from build123d import *

# Parameters (mm, degrees)
F1_DEPTH  = 16
F2_W      = 70
F2_H      = 3
F3_DEPTH  = 2
F4_W      = 50
F4_H      = 14
F5_DEPTH  = 2
F6_R      = 1
F9_DEPTH  = 2
F11_DEPTH = 38.001
F13_D     = 4
F14_R     = 3
F14_R_2   = 2
F15_DEPTH = 5
F16_R     = 3


# Not quite as in the source:
# - a pattern or mirror of a feature is missing from the dataset's text; its kind, count and spacing are read off the source's solid


with BuildPart() as f1:
    # F0 (on Front) → F1 (new body)
    with BuildSketch(Plane.XZ):
        with BuildLine():
            Line((94, 9), (0, 9))
            ThreePointArc((0, 9), (-9, 0), (0, -9))
            Line((0, -9), (19, -9))
            ThreePointArc((19, -9), (21.9483530121, -9.9617807742), (23.7624383273, -12.4771141937))
            ThreePointArc((23.7624383273, -12.4771141937), (42.5404984663, -42.5461666629), (73.3918884835, -60.0091329916))
            ThreePointArc((73.3918884835, -60.0091329916), (79.2017940664, -60.9932244785), (84.0921252778, -64.2807919045))
            Line((84.0921252778, -64.2807919045), (85.6344375761, -63))
            ThreePointArc((85.6344375761, -63), (80.1625330731, -59.2251678092), (73.628769931, -58))
            ThreePointArc((73.628769931, -58), (43.8155502437, -40.9978046119), (25.6674136582, -11.8679598712))
            ThreePointArc((25.6674136582, -11.8679598712), (23.127694217, -8.3464930839), (19, -7))
            Line((19, -7), (0, -7))
            ThreePointArc((0, -7), (-7, 0), (0, 7))
            Line((0, 7), (94, 7))
            Line((94, 7), (94, 9))
        make_face()
    extrude(amount=F1_DEPTH)

    # F2 (on face) → F3 (join)
    with BuildSketch(Plane.XY.offset(9)):
        with Locations((59, -17.5)):
            Rectangle(F2_W, F2_H)
    extrude(amount=-F3_DEPTH)

    # F4 (on face) → F5 (join)
    with BuildSketch(Plane.XZ.offset(19)):
        with Locations((69, 2)):
            Rectangle(F4_W, F4_H)
    extrude(amount=-F5_DEPTH)

    # F6
    f6_edges = [f1.edges().sort_by_distance(p)[0] for p in [
        (69, -17, 7),
        (59, -19, 9),
    ]]
    fillet(f6_edges, radius=F6_R)

    # F7: F1 across plane


with BuildPart() as f1_1:
    add(f1.part)
    add(f1.part.mirror(Plane.XZ))

    # F8 (on face) → F9 (cut)
    with BuildSketch(Plane.XY.offset(9)):
        with BuildLine():
            Line((94, 12), (34, 12))
            ThreePointArc((34, 12), (22, 0), (34, -12))
            Line((34, -12), (94, -12))
            Line((94, -12), (94, 12))
        make_face()
    extrude(amount=-F9_DEPTH, mode=Mode.SUBTRACT)

    # F10 (on face) → F11 (cut, through all)
    with BuildSketch(Plane.XZ.offset(19)):
        with BuildLine():
            ThreePointArc((50, 3), (47, 0), (50, -3))
            Line((50, -3), (70, -3))
            ThreePointArc((70, -3), (73, 0), (70, 3))
            Line((70, 3), (50, 3))
        make_face()
    extrude(amount=-F11_DEPTH, mode=Mode.SUBTRACT)

    # F13 (through all)
    with Locations(Plane.XZ.offset(19)):
        with Locations((80, 1)):
            Hole(F13_D / 2)

    # F14 (on face) → F15 (join)
    with BuildSketch(Plane(origin=(0, -17, 0), x_dir=(-1, 0, 0), z_dir=(0, 1, 0))):
        with Locations((-80, 1)):
            Circle(F14_R)
        with Locations((-80, 1)):
            Circle(F14_R_2, mode=Mode.SUBTRACT)
    f15 = extrude(amount=F15_DEPTH)

    # F15_copies: F15 across plane
    add(f15.mirror(Plane.ZX))

    # F16
    f16_edges = [f1_1.edges().sort_by_distance(p)[0] for p in [
        (94, -18, -5),
        (94, 18, -5),
        (44, 18, -5),
        (44, -18, -5),
    ]]
    fillet(f16_edges, radius=F16_R)


solid = f1_1.part
Source: CAD feature listing. Evaluate the final solid. Frame: model axes, mm. A direction names the side the tool comes from. Give positions to 0.01 mm unless a question says otherwise; leave off trailing zeros. Loops run counter-clockwise (first coordinate to the right, second up) from the corner with the lowest first, then second, coordinate; pieces in that order, holes last. Notation, with made-up numbers: (10.5, 76.5) -> (69.5, 76.5) arc R11 cw to (69.5, 83.5) -> close; hole circle Ø8 at (-3, 28). An arc over 180 degrees is marked (long way). Use a Markdown table: item, result. Add a question column.
1) Section query C-C, the plane z = 1. Count the separate pieces of the cut face and the enclosed holes in it, then the cut area to 3 significant figures.
2) Reachability of faces 5 (the face through (24, 18, 8)), 6 (the face through (79, 12, -1)), 7 (the face through (83, 15, 1)), 8 (the face through (73, -18, 0)), 9 (the face through (44.167, -0.224, -41.333)) from +Z, -Z, +X, -X, +Y, -Y: full face, straight path, thin tool, end or side. Return the list, or none.
3) Section query A-A, the plane x = 37. Return the cut outline in (y, z).
4) Line query: line 1 along Z through (x, y) = (11.5, -3); line 2 along Z through (x, y) = (55, 17.5); line 3 along Y through (x, z) = (67, 6). Output: solid intervals per line, ascending. Write a range as [from, to].
5) Section query D-D, the plane y = -6.5. Return the cut outline in (x, z), then the cut area to 3 significant figures.
6) Pull-direction query (Y, two-part tool) for faces 1 (the face through (42.18, -0.22, -42.2)), 2 (the face through (28, 16, -19)), 3 (the face through (79, -12, -1)), 4 (the face through (69, 17, 4)); classes: +Y half, -Y half, draft (parallel to the pull), parting line (faces both ways), or undercut.
7) Section query B-B, the plane y = 0. Return the cut outline in (x, z), then the cut area to 3 significant figures.
8) First-contact query: pin 1 (3 mm diameter, centred on y = -13, z = -40.5, fed in from +X); pin 2 (5 mm diameter, centred on x = 20, y = 3, fed in from -Z); pin 3 (8 mm diameter, centred on y = -10, z = -19.5, fed in from -X); pin 4 (3.5 mm diameter, centred on x = 80, z = 1, fed in from -Y). Flat tips, straight axial feed; report the tip coordinate or a pass-through.
Numbers:
| question | item | result |
|---|---|---|
| 1 | separate pieces | 7 |
| 1 | enclosed holes | 0 |
| 1 | area | 166 mm2 |
| 2 | face 5 | +Z, -Z, -X, +Y |
| 2 | face 6 | +Z, +X |
| 2 | face 7 | none |
| 2 | face 8 | +Y, -Y |
| 2 | face 9 | +X, +Y, -Y |
| 3 | outline | (-19, 7) -> (-12, 7) -> (-12, 9) -> (-18, 9) arc R1 ccw to (-19, 8) -> close; (-16, -36.61) -> (16, -36.61) -> (16, -33.41) -> (-16, -33.41) -> close; (12, 7) -> (19, 7) -> (19, 8) arc R1 ccw to (18, 9) -> (12, 9) -> close |
| 4 | line 1 | z = [-9, -7], [7, 9] |
| 4 | line 2 | z = [-5, -3], [3, 9] |
| 4 | line 3 | y = [-19, -17], [17, 19] |
| 5 | outline | (0, -9) -> (19, -9) arc R5 cw to (23.76, -12.48) arc R72 ccw to (73.39, -60.01) arc R14 cw to (84.09, -64.28) -> (85.63, -63) arc R16 ccw to (73.63, -58) arc R70 cw to (25.67, -11.87) arc R7 ccw to (19, -7) -> (0, -7) arc R7 cw to (0, 7) -> (23.91, 7) -> (23.91, 9) -> (0, 9) arc R9 ccw to start |
| 5 | area | 317 mm2 |
| 6 | face 1 | draft |
| 6 | face 2 | +Y half |
| 6 | face 3 | undercut |
| 6 | face 4 | undercut |
| 7 | outline | (0, -9) -> (19, -9) arc R5 cw to (23.76, -12.48) arc R72 ccw to (73.39, -60.01) arc R14 cw to (84.09, -64.28) -> (85.63, -63) arc R16 ccw to (73.63, -58) arc R70 cw to (25.67, -11.87) arc R7 ccw to (19, -7) -> (0, -7) arc R7 cw to (0, 7) -> (22, 7) -> (22, 9) -> (0, 9) arc R9 ccw to start |
| 7 | area | 314 mm2 |
| 8 | pin 1 | stops at x = 44.88 |
| 8 | pin 2 | stops at z = -10.43 |
| 8 | pin 3 | stops at x = 24.8 |
| 8 | pin 4 | passes through |
